Here's the drawing with two shaded views (mm, measured from the low corner). I have some questions. Give positions to 0.01 mm unless a question says otherwise; leave off trailing zeros. Order: outer loops, then holes, each group sorted by start corner. A loop starts at its lowest first (then second) coordinate and runs counter-clockwise, first axis right, second up. Notation, with made-up numbers: M 48.5,85.5 L 71.5,85.5 A31 ccw 71.5,115.5 Z; hole C 16.25,7.25 d5. An arc over 180 degrees is marked long. Use a Markdown table: item, result. Add a question column.
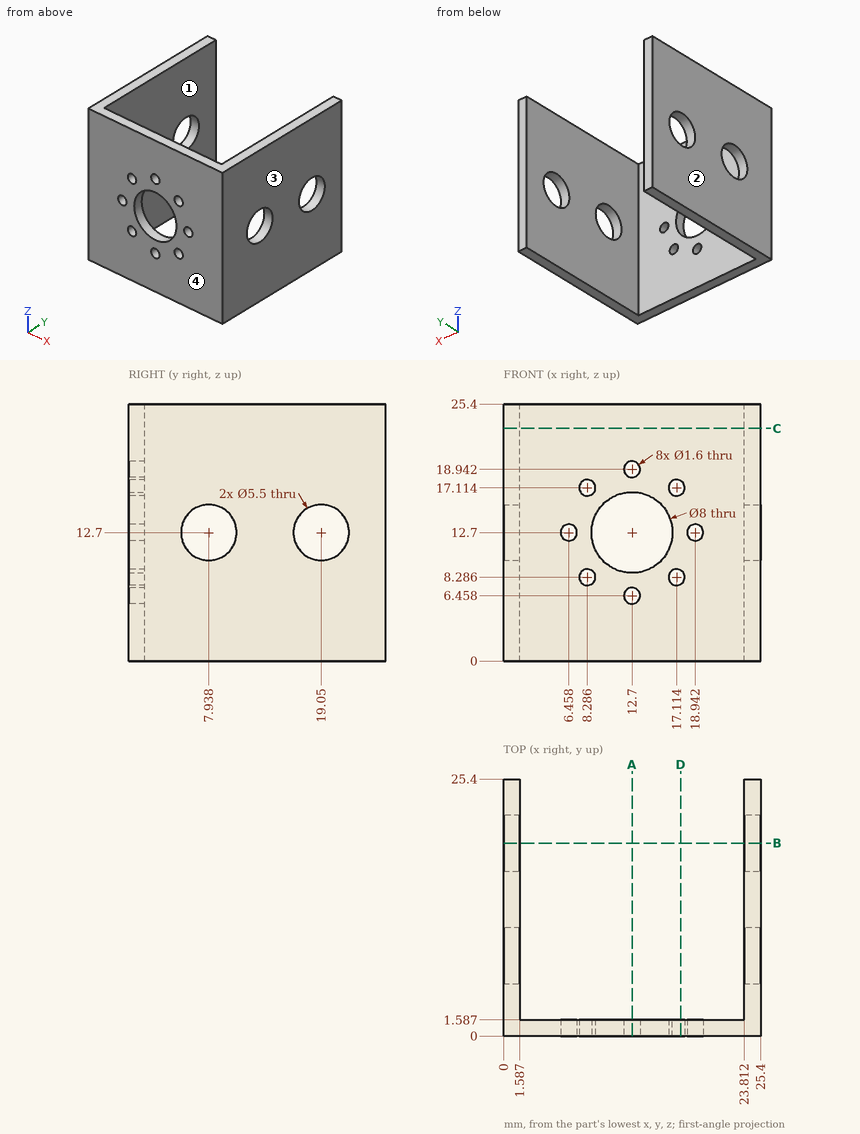
1. If we section it at A-A, the plane x = 12.7: List the corners of the cut face in (y, z) for me.
2. If we section it at B-B, the plane y = 19.05: List the corners of the cut face in (x, z) for me.
3. If we section it at D-D, the plane x = 17.5: List the corners of the cut face in (y, z) for me.
4. If we section it at C-C, the plane z = 23: List the corners of the cut face in (x, y) for me.
5. Will this pin go through, and if not, where does the flat tip stop? pin 1 (2 mm diameter, centred on x = 17.11, z = 8.29, fed in from +Y).
6. I need wall thicknesses on L1, parallel to X at y = 23.25, z = 10.75; L2, parallel to Z at x = 12.7, y = 0.95; L3, parallel to Z at x = 24.5, y = 19.05. Which ranges of each line are inside material? Lowest first, please. Write a range as [from, to].
7. We'd pull the mould along X, two halves only. Please class the marked faces 1, 2, 3 and 4: +X half, -X half, draft (parallel to the pull), parting line (faces both ways), or undercut.
Geometry results:
| question | item | result |
|---|---|---|
| 1 | outline | M 0,0 L 1.59,0 L 1.59,5.66 L 0,5.66 Z; M 0,7.26 L 1.59,7.26 L 1.59,8.7 L 0,8.7 Z; M 0,16.7 L 1.59,16.7 L 1.59,18.14 L 0,18.14 Z; M 0,19.74 L 1.59,19.74 L 1.59,25.4 L 0,25.4 Z |
| 2 | outline | M 0,0 L 1.59,0 L 1.59,9.95 L 0,9.95 Z; M 0,15.45 L 1.59,15.45 L 1.59,25.4 L 0,25.4 Z; M 23.81,0 L 25.4,0 L 25.4,9.95 L 23.81,9.95 Z; M 23.81,15.45 L 25.4,15.45 L 25.4,25.4 L 23.81,25.4 Z |
| 3 | outline | M 0,0 L 1.59,0 L 1.59,7.59 L 0,7.59 Z; M 0,8.99 L 1.59,8.99 L 1.59,16.41 L 0,16.41 Z; M 0,17.81 L 1.59,17.81 L 1.59,25.4 L 0,25.4 Z |
| 4 | outline | M 0,0 L 25.4,0 L 25.4,25.4 L 23.81,25.4 L 23.81,1.59 L 1.59,1.59 L 1.59,25.4 L 0,25.4 Z |
| 5 | pin 1 | stops at y = 1.59 |
| 6 | L1 | x = [0, 1.59], [23.81, 25.4] |
| 6 | L2 | z = [0, 5.66], [7.26, 8.7], [16.7, 18.14], [19.74, 25.4] |
| 6 | L3 | z = [0, 9.95], [15.45, 25.4] |
| 7 | face 1 | undercut |
| 7 | face 2 | -X half |
| 7 | face 3 | +X half |
| 7 | face 4 | draft |
